```python
from build123d import *

# Parameters (mm, degrees)
F0_R            = 8
F1_DEPTH        = 20
F2_R            = 5
F3_DEPTH        = 20
F5_DEPTH        = 16
F5_COPIES_COUNT = 3
F6_SIZE         = 0.49999
F7_R            = 0.5
F9_D            = 6.35
F9_DEPTH        = 14
F9_TIP          = 1.9077324654
F10_R           = 2.1
F11_DEPTH       = 8.25
F12_SIZE        = 3


# Not quite as in the source:
# - a fillet or chamfer is up to 0.001 mm smaller than in the source, because OpenCascade refuses the exact size
# - a pattern or mirror of a feature is missing from the dataset's text; its kind, count and spacing are read off the source's solid


with BuildPart() as f1:
    # F0 (on Front) → F1 (new body)
    with BuildSketch(Plane.XZ):
        Circle(F0_R)
    extrude(amount=-F1_DEPTH)

    # F2 (on face) → F3 (join)
    with BuildSketch(Plane(origin=(0, 20, 0), x_dir=(-1, 0, 0), z_dir=(0, 1, 0))):
        Circle(F2_R)
    extrude(amount=F3_DEPTH)

    # F4 (on face) → F5 (cut)
    with BuildSketch(Plane(origin=(0, 40, 0), x_dir=(-1, 0, 0), z_dir=(0, 1, 0))):
        with BuildLine():
            ThreePointArc((2.1794494718, 4.5), (0, 5), (-2.1794494718, 4.5))
            Line((-2.1794494718, 4.5), (2.1794494718, 4.5))
        make_face()
    f5 = extrude(amount=-F5_DEPTH, mode=Mode.SUBTRACT)

    # F5_copies: F5 ×3 about axis
    f5_copies_axis = Axis((0, 0, 0), (0, 1, 0))
    for i in range(1, F5_COPIES_COUNT):
        add(f5.rotate(f5_copies_axis, i * 360 / F5_COPIES_COUNT), mode=Mode.SUBTRACT)

    # F6 (size 0.5 in the source; OpenCascade refuses exactly that, so slightly less here)
    f6_edges = [f1.edges().sort_by_distance(p)[0] for p in [
        (4.330127, 40, 2.5),
        (-4.996709, 40, -0.18139),
        (0, 40, -5),
        (-4.236582, 40, 2.655443),
    ]]
    chamfer(f6_edges, length=F6_SIZE)

    # F7
    f7_edges = [f1.edges().sort_by_distance(p)[0] for p in [
        (-8, 20, 0),
        (5, 20, 0),
    ]]
    fillet(f7_edges, radius=F7_R)

    # F9
    with Locations(Plane.XZ):
        with Locations((0, 0)):
            Hole(F9_D / 2, depth=F9_DEPTH)
            with Locations((0, 0, -(F9_DEPTH + F9_TIP / 2))):  # 118° drill point
                Cone(0, F9_D / 2, F9_TIP, mode=Mode.SUBTRACT)

    # F10 (on Right) → F11 (cut, symmetric)
    with BuildSketch(Plane.YZ):
        with Locations((10, 0)):
            Circle(F10_R)
    extrude(amount=F11_DEPTH, both=True, mode=Mode.SUBTRACT)

    # F12
    f12_edges = [f1.edges().sort_by_distance(p)[0] for p in [
        (-8, 0, 0),
    ]]
    chamfer(f12_edges, length=F12_SIZE)


solid = f1.part
```
Design review of the part built by this model. Coordinates are the model's own, in mm. A direction names the side the tool comes from. Round coordinates to 2 decimals unless told otherwise and drop trailing zeros. Order: outer loops, then holes, each group sorted by start corner. A loop starts at its lowest first (then second) coordinate and runs counter-clockwise, first axis right, second up. Notation, with made-up numbers: M -27.5,-8 L -0.5,-8 A6 cw -0.5,0 Z; hole C -12,-5 d7. An arc over 180 degrees is marked long. Put each result on its own line as item: value.
Q1. To check wall thickness, follow line 1 (Y direction, x = 3.85, z = 0); line 2 (Z direction, x = -4, y = 10); line 3 (X direction, y = 4, z = 0) (3 decimals). State the ranges of each line that lie inside material, in increasing order.
Reported:
line 1: 0 to 7.9, 12.1 to 40
line 2: -6.93 to -2.1, 2.1 to 6.93
line 3: -8 to -3.175, 3.175 to 8
Q2. Consider section A-A (y = 10). State the section outline as (x, z) points (3 decimals), and give its area (3 significant figures).
Reported:
outline: M -7.719,-2.1 A8 ccw 7.719,-2.1 L 2.381,-2.1 A3.175 cw -2.381,-2.1 Z; M -7.719,2.1 L -2.381,2.1 A3.175 cw 2.381,2.1 L 7.719,2.1 A8 ccw Z
area: 128 mm²
Q3. Draft analysis for pull direction X (two halves, no side actions). For faces 1 (the face through (-4.05, 39.86, 2.26)), 2 (the face through (0.526, 15.576, 0.166)), 3 (the face through (-4.1, 24, -2.3)), state which applies: released by +X, released by -X, zero draft, split by the parting line, or undercut.
Reported:
face 1: released by -X
face 2: undercut
face 3: zero draft
Q4. Consider section B-B (y = 21.5). State the section outline as (x, z) points, and give its area (3 significant figures).
Reported:
outline: C 0,0 d10
area: 78.5 mm²
Q5. Consider section C-C (z = -0.75). State how many separate pieces and enclosed holes the cut face has, and give its area (3 significant figures).
Reported:
separate pieces: 3
enclosed holes: 0
area: 372 mm²
Q6. Machinability: for faces 4 (the face through (0, 32, 4.5)), 5 (the face through (4.1, 24, -2.4)), 6 (the face through (-4, 20, 4)), 7 (the face through (3.17, 7.1, 0.14)), which of the approach directions +Z, -Z, +X, -X, +Y, -Y give a long, thin tool a straight path to every point of the face, cutting with its end or side? Answer none if there is none.
Reported:
face 4: +Z, +X, -X, +Y
face 5: -Z, +X, +Y
face 6: +Y
face 7: -Y
Q7. Insertion check: pin 1 Ø4 at (x, z) = (0, 0) entering from -Y; pin 2 Ø1 at (x, y) = (2.5, 27) entering from -Z; pin 3 Ø3.5 at (y, z) = (10, 0) entering from +X; pin 4 Ø3 at (x, y) = (2.5, 14.5) entering from -Z. Each pin has a flat end and moves straight along its axis. Give the tip position at first contact, or say it passes through.
Reported:
pin 1: y = 14.71
pin 2: z = -4.58
pin 3: through
pin 4: z = -7.94
